The listing builds one solid part. Answer for the finished solid, in the listing's coordinates (mm). A direction names the side the tool comes from. Round coordinates to 2 decimals unless told otherwise and drop trailing zeros. Write each loop counter-clockwise with the first axis right and the second up, starting at its lowest first coordinate (ties: lowest second). Pieces come first, ordered by that corner, then holes.
Item 1: A tool of negligible diameter and unlimited length cuts with its end or side. For faces 1 (the face through (0, 14, 0)), 2 (the face through (3.905, 0.493, 0.867)), 3 (the face through (4.88, 12.27, 1.08)), from which of +Z, -Z, +X, -X, +Y, -Y can it reach the whole face along a straight path? Write none if from no direction.
Item 2: Find section C-C on y = 9.75. Give the vertices of the cut face in (x, z).
Item 3: Each of these flat-tipped pins is pushed along its axis until it touches: pin 1 (1.5 mm diameter, centred on x = -3, y = 3.5, fed in from +Z); pin 2 (3 mm diameter, centred on x = 2.5, y = 12.5, fed in from -Z); pin 3 (1 mm diameter, centred on y = 13, z = 3.5, fed in from +X). Where does it stop, or does it pass through?
Item 4: Find section D-D on y = 11.75. Give the vertices of the cut face in (x, z), then the cut area to 3 significant figures.
Item 5: Find the intervals of material crossed by probe 1 along X at (y, z) = (0.4, 0); probe 2 along Y at (x, z) = (3.75, 2.75); probe 3 along Y at (x, z) = (1.25, 1.25), in increasing order.
Item 6: For a pull along Z with two mould halves and no side action, classify faces 4 (the face through (4.88, 0.99, 1.08)), 5 (the face through (3.417, 5.936, 0.759)), 6 (the face through (0, 15, 0)) as +Z half, -Z half, draft (parallel to the pull), parting line (faces both ways), or undercut.
```python
from build123d import *

# Parameters (mm, degrees)
SHELL4_T  = -1
FILLET1_R = 0.4
FILLET2_R = 0.4
FILLET3_R = 0.4


with BuildPart() as part:
    # Sketch1 → Revolve2 (revolve)
    with BuildSketch(Plane.XY, mode=Mode.PRIVATE) as revolve2_sk:
        Polygon((0, 15), (-5, 15), (-5, 10), (-4.5, 10), (-4.5, 2), (-5, 2), (-5, 0), (0, 0), align=None)
    revolve(revolve2_sk.sketch.rotate(Axis((0, 0, 0), (0, 1, 0)), 270), axis=Axis((0, 0, 0), (0, 1, 0)))

    # Shell4
    shell4_openings = [part.faces().sort_by_distance(p)[0] for p in [
        (0, 0, 0),
    ]]
    offset(amount=SHELL4_T, openings=shell4_openings, kind=Kind.INTERSECTION)

    # Fillet1
    fillet1_edges = [part.edges().sort_by_distance(p)[0] for p in [
        (0, 15, 5),
    ]]
    fillet(fillet1_edges, radius=FILLET1_R)

    # Fillet2
    fillet2_edges = [part.edges().sort_by_distance(p)[0] for p in [
        (0, 1, 3.5),
    ]]
    fillet(fillet2_edges, radius=FILLET2_R)

    # Fillet3
    fillet3_edges = [part.edges().sort_by_distance(p)[0] for p in [
        (0, 11, 3.5),
    ]]
    fillet(fillet3_edges, radius=FILLET3_R)


solid = part.part
```
Check values:
1. face 1: none
1. face 2: -Y
1. face 3: +Y, -Y
2. outline: circle Ø9 at (0, 0); hole circle Ø7 at (0, 0)
3. pin 1: stops at z = 3.9
3. pin 2: stops at z = -4.9
3. pin 3: stops at x = 4
4. outline: circle Ø10 at (0, 0); hole circle Ø8 at (0, 0)
4. area: 28.3 mm2
5. probe 1: x = -5 to -4, 4 to 5
5. probe 2: y = 0 to 2, 10 to 15
5. probe 3: y = 14 to 15
6. face 4: parting line
6. face 5: undercut
6. face 6: draft
